Check sheet for the modelled part. Datum: model origin and axes. Units: mm. A direction names the side the tool comes from. Round coordinates to 2 decimals unless told otherwise and drop trailing zeros. Loops run counter-clockwise (first coordinate to the right, second up) from the corner with the lowest first, then second, coordinate; pieces in that order, holes last. Notation, with made-up numbers: (-15, -3.5) - (33, -3.5) arc R13 ccw to (33, 10.5) - close; hole circle Ø4 at (-10, -25). An arc over 180 degrees is marked (long way). Put each result on its own line as item: value.
```python
from build123d import *

# Parameters (mm, degrees)
SKETCH1_W             = 85.598
SKETCH1_H             = 50.8
BOSS_EXTRUDE1_DEPTH   = 2.159
SKETCH2_W             = 85.598
SKETCH2_H             = 2.159
BOSS_EXTRUDE2_DEPTH   = 9.271
FILLET1_R             = 1.27
FILLET2_R             = 1.27
FILLET3_R             = 2.54
FILLET4_R             = 7.62
SKETCH3_W             = 57.15
SKETCH3_H             = 25.4
CUT_EXTRUDE1_DEPTH    = 3.159
FILLET5_R             = 5.08
F_4_CLEARANCE_HOLE1_D = 3.2639
SKETCH6_R             = 3.81
BOSS_EXTRUDE3_DEPTH   = 3.048
SKETCH8_R             = 1.9685
CUT_EXTRUDE2_DEPTH    = 3.429
SKETCH9_R             = 0.9525
CUT_EXTRUDE3_DEPTH    = 2.778


with BuildPart() as part:
    # Sketch1 → Boss-Extrude1 (new body)
    with BuildSketch(Plane.XY):
        Rectangle(SKETCH1_W, SKETCH1_H)
    extrude(amount=BOSS_EXTRUDE1_DEPTH)

    # Sketch2 → Boss-Extrude2 (add)
    with BuildSketch(Plane.XY.offset(2.159)):
        with Locations((0, 24.3205)):
            Rectangle(SKETCH2_W, SKETCH2_H)
    extrude(amount=BOSS_EXTRUDE2_DEPTH)

    # Fillet1
    fillet1_edges = [part.edges().sort_by_distance(p)[0] for p in [
        (0, 23.241, 2.159),
    ]]
    fillet(fillet1_edges, radius=FILLET1_R)

    # Fillet2
    fillet2_edges = [part.edges().sort_by_distance(p)[0] for p in [
        (0, 25.4, 0),
    ]]
    fillet(fillet2_edges, radius=FILLET2_R)

    # Fillet3
    fillet3_edges = [part.edges().sort_by_distance(p)[0] for p in [
        (42.799, 24.3205, 11.43),
        (-42.799, 24.3205, 11.43),
    ]]
    fillet(fillet3_edges, radius=FILLET3_R)

    # Fillet4
    fillet4_edges = [part.edges().sort_by_distance(p)[0] for p in [
        (42.799, -25.4, 1.0795),
        (-42.799, -25.4, 1.0795),
    ]]
    fillet(fillet4_edges, radius=FILLET4_R)

    # Sketch3 → Cut-Extrude1 (cut, through all)
    with BuildSketch(Plane.XY.offset(2.159)):
        with Locations((-2.286, -0.762)):
            Rectangle(SKETCH3_W, SKETCH3_H)
    extrude(amount=-CUT_EXTRUDE1_DEPTH, mode=Mode.SUBTRACT)

    # Fillet5
    fillet5_edges = [part.edges().sort_by_distance(p)[0] for p in [
        (-30.861, -13.462, 1.0795),
        (-30.861, 11.938, 1.0795),
        (26.289, 11.938, 1.0795),
        (26.289, -13.462, 1.0795),
    ]]
    fillet(fillet5_edges, radius=FILLET5_R)

    # #4 Clearance Hole1 (through all)
    with Locations(Plane(origin=(0, 23.241, 0), x_dir=(-1, 0, 0), z_dir=(0, -1, 0))):
        with Locations((-38.1, -7.62), (24.13, -7.62)):
            Hole(F_4_CLEARANCE_HOLE1_D / 2)

    # Sketch6 → Boss-Extrude3 (add)
    with BuildSketch(Plane.XY.offset(2.159)):
        with Locations((35.179, -1.27)):
            Circle(SKETCH6_R)
        with Locations((-37.44214, 6.4262)):
            Circle(SKETCH6_R)
    extrude(amount=BOSS_EXTRUDE3_DEPTH)

    # Sketch8 → Cut-Extrude2 (cut)
    with BuildSketch(Plane.XY.offset(5.207)):
        with Locations((-37.44214, 6.4262)):
            Circle(SKETCH8_R)
        with Locations((35.179, -1.27)):
            Circle(SKETCH8_R)
    extrude(amount=-CUT_EXTRUDE2_DEPTH, mode=Mode.SUBTRACT)

    # Sketch9 → Cut-Extrude3 (cut, through all)
    with BuildSketch(Plane.XY.offset(1.778)):
        with Locations((-37.44214, 6.4262)):
            Circle(SKETCH9_R)
        with Locations((35.179, -1.27)):
            Circle(SKETCH9_R)
    extrude(amount=-CUT_EXTRUDE3_DEPTH, mode=Mode.SUBTRACT)


solid = part.part
```
Item 1: Tool access check on faces 4 (the cylindrical face through (39.657, 24.336, 7.13)), 5 (the cylindrical face through (38.7, -2.73, 3.66)), 6 (the flat face through (-30.861, -1, 1)), 7 (the flat face through (-35.8, 4.8, 5.207)). Record the directions out of +Z, -Z, +X, -X, +Y, -Y that give a thin tool (end or side, any length) a straight path to the whole face; none if there is none.
Filled sheet:
face 4: +Y, -Y
face 5: +Z
face 6: +Z, -Z
face 7: +Z, +X, -X, -Y
Item 2: Section check B-B on y = -1.27. Enter the section's corners in (x, z), then the cut area to 3 significant figures.
Filled sheet:
outline: (-42.8, 0) - (-30.86, 0) - (-30.86, 2.16) - (-42.8, 2.16) - close; (26.29, 0) - (34.23, 0) - (34.23, 1.78) - (33.21, 1.78) - (33.21, 5.21) - (31.37, 5.21) - (31.37, 2.16) - (26.29, 2.16) - close; (36.13, 0) - (42.8, 0) - (42.8, 2.16) - (38.99, 2.16) - (38.99, 5.21) - (37.15, 5.21) - (37.15, 1.78) - (36.13, 1.78) - close
area: 67.8 mm²
Item 3: Section check C-C on z = 7.62. Enter the section's corners in (x, y), then the cut area to 3 significant figures.
Filled sheet:
outline: (-42.8, 23.24) - (-25.76, 23.24) - (-25.76, 25.4) - (-42.8, 25.4) - close; (-22.5, 23.24) - (36.47, 23.24) - (36.47, 25.4) - (-22.5, 25.4) - close; (39.73, 23.24) - (42.8, 23.24) - (42.8, 25.4) - (39.73, 25.4) - close
area: 171 mm²
Item 4: Go/stop test with flat-tipped pins: pin 1 (6.5 mm diameter, centred on x = 35.179, y = -1.27, fed in from -Z); pin 2 (3 mm diameter, centred on y = -19.5, z = 2.5, fed in from -X); pin 3 (4 mm diameter, centred on x = 34, y = -3, fed in from +Z); pin 4 (2.5 mm diameter, centred on x = -37.44, y = 6.43, fed in from +Z). Record where each tip stops, or that it passes through.
Filled sheet:
pin 1: z = 0
pin 2: x = -42.79
pin 3: z = 5.21
pin 4: z = 1.78
Item 5: Section check D-D on x = -24.13. Enter the section's corners in (y, z), then the cut area to 3 significant figures.
Filled sheet:
outline: (-25.4, 0) - (-13.46, 0) - (-13.46, 2.16) - (-25.4, 2.16) - close; (11.94, 0) - (24.13, 0) arc R1.27 ccw to (25.4, 1.27) - (25.4, 5.99) - (23.24, 5.99) - (23.24, 3.43) arc R1.27 cw to (21.97, 2.16) - (11.94, 2.16) - close; (23.24, 9.25) - (25.4, 9.25) - (25.4, 11.43) - (23.24, 11.43) - close
area: 67.8 mm²
Item 6: Release check for a two-part mould opening along X. For faces 1 (the flat face through (42.799, 5, 1)), 2 (the flat face through (0, -25.4, 1)), 3 (the flat face through (-3, 11.938, 1)) record: +X half, -X half, draft (parallel to the pull), parting line (faces both ways), or undercut.
Filled sheet:
face 1: +X half
face 2: draft
face 3: undercut
Item 7: Thickness scan on line 1 (X direction, y = 24.2, z = 7.62); line 2 (Z direction, x = -24.13, y = 24.25); line 3 (X direction, y = -1, z = 4.5). Record the ranges inside material, lowest first. Write a range as from..to.
Filled sheet:
line 1: -42.8..-25.76, -22.5..36.47, 39.73..42.8
line 2: 0.01..5.99, 9.25..11.43
line 3: 31.38..33.23, 37.13..38.98
Item 8: Section check A-A on x = -2. Enter the section's corners in (y, z), then the cut area to 3 significant figures.
Filled sheet:
outline: (-25.4, 0) - (-13.46, 0) - (-13.46, 2.16) - (-25.4, 2.16) - close; (11.94, 0) - (24.13, 0) arc R1.27 ccw to (25.4, 1.27) - (25.4, 11.43) - (23.24, 11.43) - (23.24, 3.43) arc R1.27 cw to (21.97, 2.16) - (11.94, 2.16) - close
area: 74.9 mm²
